```python
from build123d import *

# Parameters (mm, degrees)
SM_BASE_FLANGE_1_DEPTH      = 32.5
HOLE_WIZARD_M4_1_D          = 3.3
HOLE_WIZARD_M4_1_DEPTH      = 11.5
HOLE_WIZARD_M4_1_TIP        = 0.991420021
OTHER_START                 = -32.5
OTHER_1_DEPTH               = 65
OTHER_1_2_DEPTH             = 65
CUT_EXTRUDE_1_REACH         = 79.484
SKETCH_11_W                 = 41
SKETCH_11_H                 = 27
OTHER_1_3_DEPTH             = 65
OTHER_1_3_2_DEPTH           = 65
HOLE_WIZARD_4_5_4_5_1_D     = 4.5
HOLE_WIZARD_4_5_4_5_1_DEPTH = 2.5
CHAMFER_1_SIZE              = 1


# Read off the part's stored shape, not the designer's step: 展开1, 折叠1
# Sheet-metal steps are written as plain solids
with BuildPart() as part:
    # Sketch 1 → 基体-法兰1 (new, symmetric)
    with BuildSketch(Plane(origin=(0, 0, 0), x_dir=(0, 0, -1), z_dir=(1, 0, 0))):
        with BuildLine():
            Line((-22.5, 32), (-22.5, 3.2366))
            ThreePointArc((-22.5, 3.2366), (-21.552021808, 0.947978192), (-19.2634, 0))
            Line((-19.2634, 0), (19.2634, 0))
            ThreePointArc((19.2634, 0), (21.552021808, 0.947978192), (22.5, 3.2366))
            Line((22.5, 3.2366), (22.5, 32))
            Line((22.5, 32), (20, 32))
            Line((20, 32), (20, 3.2366))
            ThreePointArc((20, 3.2366), (19.784254855, 2.715745145), (19.2634, 2.5))
            Line((19.2634, 2.5), (-19.2634, 2.5))
            ThreePointArc((-19.2634, 2.5), (-19.784254855, 2.715745145), (-20, 3.2366))
            Line((-20, 3.2366), (-20, 32))
            Line((-20, 32), (-22.5, 32))
        make_face()
    extrude(amount=SM_BASE_FLANGE_1_DEPTH, both=True)

    # M4 螺纹孔1
    with Locations(Plane(origin=(0, 6, 22.5), x_dir=(1, 0, 0), z_dir=(0, 0, 1))):
        with Locations((-24.315, 14.75), (-24.315, 4.75), (24.315, 14.75), (24.315, 4.75)):
            Hole(HOLE_WIZARD_M4_1_D / 2, depth=HOLE_WIZARD_M4_1_DEPTH)
            with Locations((0, 0, -(HOLE_WIZARD_M4_1_DEPTH + HOLE_WIZARD_M4_1_TIP / 2))):  # 118° drill point
                Cone(0, HOLE_WIZARD_M4_1_D / 2, HOLE_WIZARD_M4_1_TIP, mode=Mode.SUBTRACT)

    # Other 1 outline → Other 1 (cut)
    with BuildSketch(Plane.YZ.offset(OTHER_START)):
        with BuildLine():
            Line((3.2366, 20), (0.084933774, 20))
            ThreePointArc((0.084933774, 20), (0.021303554, 19.634140241), (0, 19.2634))
            Line((0, 19.2634), (0, -19.2634))
            ThreePointArc((0, -19.2634), (0.947978192, -21.552021808), (3.2366, -22.5))
            Line((3.2366, -22.5), (32, -22.5))
            Line((32, -22.5), (32, -20))
            Line((32, -20), (3.2366, -20))
            ThreePointArc((3.2366, -20), (2.715745145, -19.784254855), (2.5, -19.2634))
            Line((2.5, -19.2634), (2.5, 19.2634))
            ThreePointArc((2.5, 19.2634), (2.715745145, 19.784254855), (3.2366, 20))
        make_face()
    extrude(amount=OTHER_1_DEPTH, mode=Mode.SUBTRACT)

    # Other 1 2 outline → Other 1 2 (add)
    with BuildSketch(Plane.YZ.offset(OTHER_START)):
        with BuildLine():
            Line((3.2366, 22.5), (-70.294687966, 22.5))
            Line((-70.294687966, 22.5), (-70.294687966, 20))
            Line((-70.294687966, 20), (0.084933774, 20))
            ThreePointArc((0.084933774, 20), (1.225195018, 21.799110859), (3.2366, 22.5))
        make_face()
    extrude(amount=OTHER_1_2_DEPTH)

    # 草图11 → 切除-拉伸1 (cut, up to next)
    with BuildSketch(Plane(origin=(0, 0, 20), x_dir=(-1, 0, 0), z_dir=(0, 0, -1)), mode=Mode.PRIVATE) as cut_extrude_1_sk1:
        with Locations((0, 18.5)):
            Rectangle(SKETCH_11_W, SKETCH_11_H)
    cut_extrude_1_tool1 = extrude(cut_extrude_1_sk1.sketch, amount=-CUT_EXTRUDE_1_REACH, mode=Mode.PRIVATE) & part.part
    add(cut_extrude_1_tool1.solids().sort_by_distance((0, 18.5, 20))[0], mode=Mode.SUBTRACT)

    # Other 1 3 outline → Other 1 3 (cut)
    with BuildSketch(Plane.YZ.offset(OTHER_START)):
        with BuildLine():
            Line((-70.294687966, 20), (0.084933774, 20))
            ThreePointArc((0.084933774, 20), (1.225195018, 21.799110859), (3.2366, 22.5))
            Line((3.2366, 22.5), (-70.294687966, 22.5))
            Line((-70.294687966, 22.5), (-70.294687966, 20))
        make_face()
    extrude(amount=OTHER_1_3_DEPTH, mode=Mode.SUBTRACT)

    # Other 1 3 2 outline → Other 1 3 2 (add)
    with BuildSketch(Plane.YZ.offset(OTHER_START)):
        with BuildLine():
            ThreePointArc((0.084933774, 20), (0.021303554, 19.634140241), (0, 19.2634))
            Line((0, 19.2634), (0, -19.2634))
            ThreePointArc((0, -19.2634), (0.947978192, -21.552021808), (3.2366, -22.5))
            Line((3.2366, -22.5), (32, -22.5))
            Line((32, -22.5), (32, -20))
            Line((32, -20), (3.2366, -20))
            ThreePointArc((3.2366, -20), (2.715745145, -19.784254855), (2.5, -19.2634))
            Line((2.5, -19.2634), (2.5, 19.2634))
            ThreePointArc((2.5, 19.2634), (2.715745145, 19.784254855), (3.2366, 20))
            Line((3.2366, 20), (0.084933774, 20))
        make_face()
    extrude(amount=OTHER_1_3_2_DEPTH)

    # Ø4.5 (4.5) 直径孔1
    with Locations(Plane(origin=(0, 0, -22.5), x_dir=(-1, 0, 0), z_dir=(0, 0, -1))):
        with Locations((-22.5, 26), (-22.5, 11), (22.5, 26), (22.5, 11)):
            Hole(HOLE_WIZARD_4_5_4_5_1_D / 2, depth=HOLE_WIZARD_4_5_4_5_1_DEPTH)

    # 倒角1
    chamfer_1_edges = [part.edges().sort_by_distance(p)[0] for p in [
        (32.5, 32, 21.25),
        (-32.5, 32, 21.25),
        (32.5, 32, -21.25),
        (-32.5, 32, -21.25),
    ]]
    chamfer(chamfer_1_edges, length=CHAMFER_1_SIZE)


solid = part.part
```
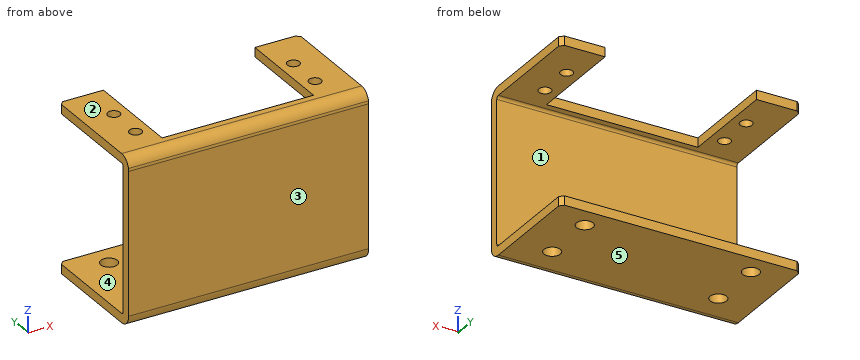
Can you work these out from the model? Positions are in its coordinate system, mm. Face numbers are marked on the shaded views. A direction names the side the tool comes from. Give positions to 0.01 mm unless a question says otherwise; leave off trailing zeros. Order: outer loops, then holes, each group sorted by start corner. A loop starts at its lowest first (then second) coordinate and runs counter-clockwise, first axis right, second up. Notation, with made-up numbers: (29, 79) - (45, 79) arc R14 cw to (45, 102) - close; hole circle Ø9 at (2.25, 13). An arc over 180 degrees is marked (long way). Use a Markdown table: item, result. Add a question column.
Q1. If we section it at B-B on x = 27: Write out the boundary of the cut face in (y, z), plus the area to 3 significant figures.
Q2. If we section it at D-D on x = -21.5: Write out the boundary of the cut face in (y, z).
Q3. I'm going to push flat-ended pins straight in: pin 1 (1.5 mm diameter, centred on x = 19.5, z = 14.5, fed in from +Y); pin 2 (2 mm diameter, centred on x = -3.5, z = 22, fed in from +Y); pin 3 (2 mm diameter, centred on x = 16, y = 28.5, fed in from +Z); pin 4 (5 mm diameter, centred on y = 5.5, z = -0.5, fed in from +X). Where does each tip first touch, or does it pass through?
Q4. If we section it at C-C on y = 29: Write out the boundary of the cut face in (x, z), plus the area to 4 significant figures.
Q5. Please list where these lines run through material, in increasing order: line 1 along Y through (x, z) = (22.5, -21.15); line 2 along Y through (x, z) = (22, -21); line 3 along Z through (x, y) = (-23.5, 25.5).
Q6. If we section it at A-A on y = 20.75: Write out the boundary of the cut face in (x, z) (3 decimals), plus the area to 3 significant figures.
Q7. On a 3-axis mill with a long thin cutter (end or side, diameter ignored), from which of +Z, -Z, +X, -X, +Y, -Y can I reach the whole of each face in a straight line? I mean the marked faces 4 and 5. Say none if no direction works.
Q8. If we mould it in two halves opening along Z, with no side actions, what happens to the marked faces 1, 2 and 3? For each: released by +Z, released by -Z, zero draft, split by the parting line, or undercut.
Answers follow:
| question | item | result |
|---|---|---|
| 1 | outline | (0, -19.26) arc R3.24 ccw to (3.24, -22.5) - (32, -22.5) - (32, -20) - (3.24, -20) arc R0.74 cw to (2.5, -19.26) - (2.5, 19.26) arc R0.74 cw to (3.24, 20) - (32, 20) - (32, 22.5) - (3.24, 22.5) arc R3.24 ccw to (0, 19.26) - close |
| 1 | area | 256 mm^2 |
| 2 | outline | (0, -19.26) arc R3.24 ccw to (3.24, -22.5) - (8.98, -22.5) - (8.98, -20) - (3.24, -20) arc R0.74 cw to (2.5, -19.26) - (2.5, 19.26) arc R0.74 cw to (3.24, 20) - (32, 20) - (32, 22.5) - (3.24, 22.5) arc R3.24 ccw to (0, 19.26) - close; (13.02, -22.5) - (23.98, -22.5) - (23.98, -20) - (13.02, -20) - close; (28.02, -22.5) - (32, -22.5) - (32, -20) - (28.02, -20) - close |
| 3 | pin 1 | stops at y = 2.5 |
| 3 | pin 2 | stops at y = 5 |
| 3 | pin 3 | stops at z = -20 |
| 3 | pin 4 | passes through |
| 4 | outline | (-32.5, -22.5) - (32.5, -22.5) - (32.5, -20) - (-32.5, -20) - close; (-32.5, 20) - (-20.5, 20) - (-20.5, 22.5) - (-32.5, 22.5) - close; (20.5, 20) - (32.5, 20) - (32.5, 22.5) - (20.5, 22.5) - close |
| 4 | area | 222.5 mm^2 |
| 5 | line 1 | y = 0.61 to 8.75, 13.25 to 23.75, 28.25 to 32 |
| 5 | line 2 | y = 0.51 to 8.81, 13.19 to 23.81, 28.19 to 32 |
| 5 | line 3 | z = 20 to 22.5 |
| 6 | outline | (-32.5, -22.5) - (32.5, -22.5) - (32.5, -20) - (-32.5, -20) - close; (-32.5, 20) - (-25.965, 20) - (-25.965, 22.5) - (-32.5, 22.5) - close; (-22.665, 20) - (-20.5, 20) - (-20.5, 22.5) - (-22.665, 22.5) - close; (20.5, 20) - (22.665, 20) - (22.665, 22.5) - (20.5, 22.5) - close; (25.965, 20) - (32.5, 20) - (32.5, 22.5) - (25.965, 22.5) - close |
| 6 | area | 206 mm^2 |
| 7 | face 4 | +X, -X, +Y |
| 7 | face 5 | -Z, +X, -X, +Y, -Y |
| 8 | face 1 | undercut |
| 8 | face 2 | released by +Z |
| 8 | face 3 | zero draft |
